Autodesk Inventor part; units mm, degrees
ref_plane "YZ Plane" through (0, 0, 0) normal (1, 0, 0) x (0, 1, 0)
ref_plane "XZ Plane" through (0, 0, 0) normal (0, 1, 0) x (-1, 0, 0)
ref_plane "XY Plane" through (0, 0, 0) normal (0, 0, 1) x (1, 0, 0)
sketch "Sketch1" plane through (0, 0, 0) normal (0, 0, 1) x (1, 0, 0)
  line L0 (0, 0) -> (22, 0)
  line L1 (22, 0) -> (22, 28)
  line L2 (22, 28) -> (0, 28)
  line L3 (0, 28) -> (0, 0)
  dimension "d0" = 22
  dimension "d1" = 28
extrude "Extrusion1" add sketch "Sketch1" along normal blind 2
sketch "Sketch2" plane through (0, 0, 2) normal (0, 0, 1) x (1, 0, 0)
  line L0 (0, 0) -> (22, 0)
  line L1 (0, 28) -> (0, 0)
  point P0 (2, 2)
  dimension "d34" = 2
  dimension "d35" = 2
hole "Hole1" at (2, 2, 2) direction (0, 0, -1) diameter 2.6 end through all
sketch "Sketch3" plane through (0, 0, 2) normal (0, 0, 1) x (1, 0, 0)
  line L0 (22, 0) -> (22, 28)
  line L1 (0, 0) -> (22, 0)
  point P0 (20, 2)
  dimension "d32" = 2
  dimension "d33" = 2
hole "Hole2" at (20, 2, 2) direction (0, 0, -1) diameter 2.6 end through all
sketch "Sketch4" plane through (0, 0, 2) normal (0, 0, 1) x (1, 0, 0)
  circle A0 centre (2, 2) radius 1.3
  line L0 (0, 28) -> (0, 0)
  point P0 (2, 13)
  dimension "d38" = 11
  dimension "d39" = 2
hole "Hole3" at (2, 13, 2) direction (0, 0, -1) diameter 2.6 end through all
sketch "Sketch5" plane through (0, 0, 2) normal (0, 0, 1) x (1, 0, 0)
  line L0 (22, 0) -> (22, 28)
  circle A0 centre (20, 2) radius 1.3
  point P0 (0, 0)
  point P1 (20, 13)
  dimension "d36" = 2
  dimension "d37" = 11
hole "Hole4" at (20, 13, 2) direction (0, 0, -1) diameter 2.6 end through all
sketch "Sketch6" plane through (0, 0, 2) normal (0, 0, 1) x (1, 0, 0)
  line L0 (8.5, 9.25) -> (13.5, 9.25)
  line L1 (13.5, 9.25) -> (13.5, 5.75)
  line L2 (13.5, 5.75) -> (8.5, 5.75)
  line L3 (8.5, 5.75) -> (8.5, 9.25)
  line L4 (0, 0) -> (22, 0)
  line L5 (0, 28) -> (0, 0)
  dimension "d40" = 5
  dimension "d41" = 3.5
  dimension "d42" = 5.75
  dimension "d43" = 8.5
extrude "Extrusion2" add sketch "Sketch6" along normal blind 1
properties part number "angle hall sensor"
Here's how the part is built. I have some questions about the finished solid (model axes, mm). A direction names the side the tool comes from. Give positions to 0.01 mm unless a question says otherwise; leave off trailing zeros. Loops run counter-clockwise (first coordinate to the right, second up) from the corner with the lowest first, then second, coordinate; pieces in that order, holes last. Notation, with made-up numbers: (54, 89) -> (97, 89) arc R14 ccw to (97, 113) -> close; hole circle Ø5 at (36.25, 44.5). An arc over 180 degrees is marked (long way). Use one line per item in the form item = value. Start each with the question number.
1) Imagine slicing it at A-A (y = 12.5). Please give me the cut outline in (x, z).
2) Imagine slicing it at D-D (y = 8.5). Please give me the cut outline in (x, z), then the cut area to 3 significant figures.
3) Which directions (+Z, -Z, +X, -X, +Y, -Y) give clear straight access to the entire face, cutting with the end or side of a thin tool? Please do faces 1 (the face through (11, 9.25, 2.5)), 2 (the face through (11, 5.75, 2.5)), 3 (the face through (8.5, 7.5, 2.5)).
4) Thinking about a two-plate mould opening in Y: for faces 4 (the face through (11, 8, 3)), 5 (the face through (11, 0, 1)), 6 (the face through (3.27, 13.28, 0.99)), which applies, +Y half, -Y half, draft (parallel to the pull), parting line (faces both ways), or undercut?
5) Imagine slicing it at C-C (z = 0.75). Please give me the cut outline in (x, y).
6) For P1, Ø1.6, axis at x = 2, y = 13, coming from the -Z side; P2, Ø0.8, axis at y = 6.5, z = 2.5, coming from the -X side; P3, Ø3.5, axis at x = 20, y = 13, coming from the +Z side; P4, Ø12, axis at x = 18, y = 17, coming from the -Z side, each with a flat end and sliding along its axis, tell me the tip position at first contact or that it passes through.
7) Please list where these lines run through material, in increasing order: line 1 along X through (y, z) = (13, 1); line 2 along Y through (x, z) = (20, 1.35); line 3 along Z through (x, y) = (14, 24.75).
8) Imagine slicing it at B-B (x = 2.5). Please give me the cut outline in (y, z).
Check values:
q1.outline = (0, 0) -> (0.8, 0) -> (0.8, 2) -> (0, 2) -> close; (3.2, 0) -> (18.8, 0) -> (18.8, 2) -> (3.2, 2) -> close; (21.2, 0) -> (22, 0) -> (22, 2) -> (21.2, 2) -> close
q2.outline = (0, 0) -> (22, 0) -> (22, 2) -> (13.5, 2) -> (13.5, 3) -> (8.5, 3) -> (8.5, 2) -> (0, 2) -> close
q2.area = 49.0 mm^2
q3.face_1 = +Z, +X, -X, +Y
q3.face_2 = +Z, +X, -X, -Y
q3.face_3 = +Z, -X, +Y, -Y
q4.face_4 = draft
q4.face_5 = -Y half
q4.face_6 = undercut
q5.outline = (0, 0) -> (22, 0) -> (22, 28) -> (0, 28) -> close; hole circle Ø2.6 at (2, 2); hole circle Ø2.6 at (2, 13); hole circle Ø2.6 at (20, 2); hole circle Ø2.6 at (20, 13)
q6.P1 = through
q6.P2 = 8.5
q6.P3 = 2
q6.P4 = 0
q7.line_1 = 0 to 0.7, 3.3 to 18.7, 21.3 to 22
q7.line_2 = 0 to 0.7, 3.3 to 11.7, 14.3 to 28
q7.line_3 = 0 to 2
q8.outline = (0, 0) -> (0.8, 0) -> (0.8, 2) -> (0, 2) -> close; (3.2, 0) -> (11.8, 0) -> (11.8, 2) -> (3.2, 2) -> close; (14.2, 0) -> (28, 0) -> (28, 2) -> (14.2, 2) -> close
